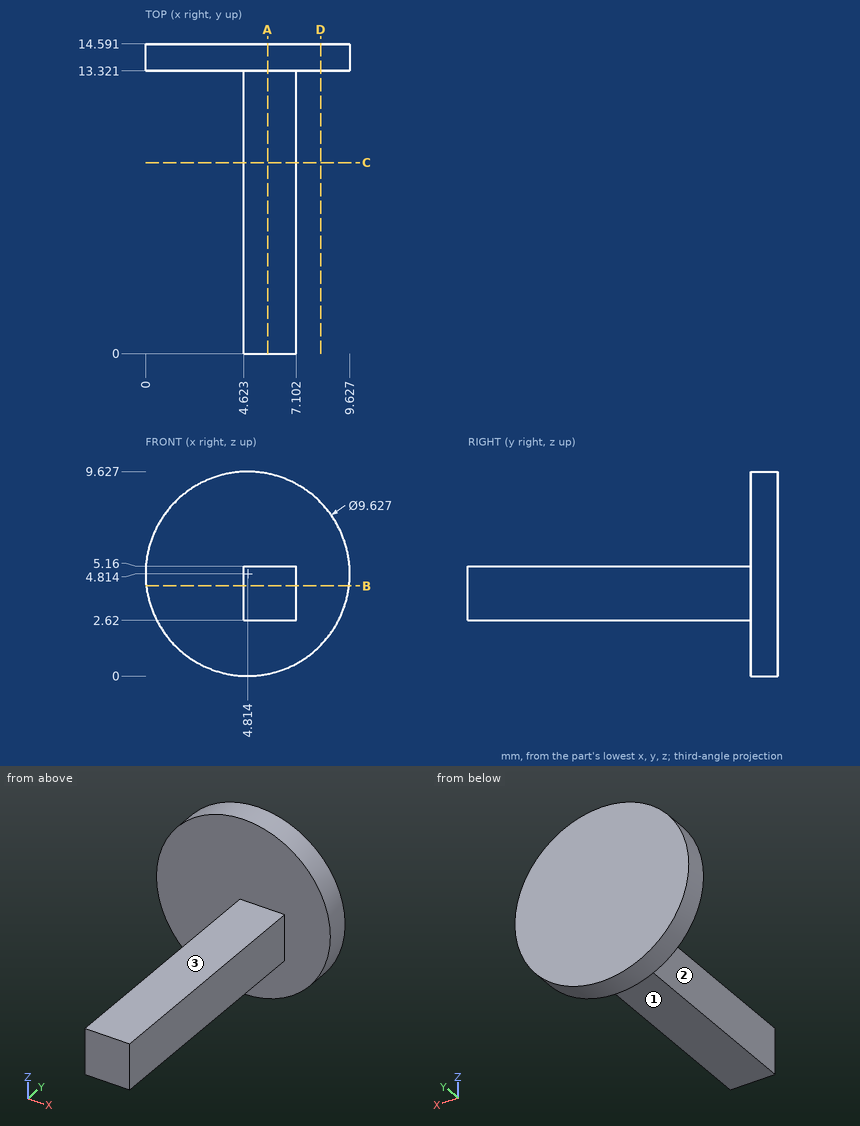
Job drawing, mm, ordinate dimensions from the low corner. One solid piece. A direction names the side the tool comes from. Round coordinates to 2 decimals unless told otherwise and drop trailing zeros. Loops run counter-clockwise (first coordinate to the right, second up) from the corner with the lowest first, then second, coordinate; pieces in that order, holes last.
Item 1: Cut at A-A, the plane x = 5.75. Give the cut face in (y, z) (1 decimal).
Item 2: Drop flat-ended pins along their axis: P1, Ø0.8, axis at y = 4.5, z = 4.5, coming from the +X side; P2, Ø2, axis at x = 6.5, y = 9, coming from the +Z side; P3, Ø4, axis at y = 7, z = 8, coming from the +X side; P4, Ø4, axis at y = 12, z = 2.5, coming from the -X side. Give the stop position or say it passes through.
Item 3: Cut at D-D, the plane x = 8.25. Give the cut face in (y, z) (1 decimal).
Item 4: 3-axis set-ups, long thin cutter, end or side, ignore diameter. For the marked faces 1, 2 and 3: which of +Z, -Z, +X, -X, +Y, -Y reach the whole face in a straight line?
Item 5: Drill centre lines: line 1 (Y direction, x = 3.5, z = 2); line 2 (X direction, y = 11.75, z = 4.75); line 3 (Z direction, x = 4.75, y = 12.5). Where is each one in solid material? Low to high.
Item 6: Cut at B-B, the plane z = 4.25. Give the cut face in (x, y) (1 decimal).
Item 7: Cut at C-C, the plane y = 9. Give the cut face in (x, z).
A:
1. outline: (0, 2.6) - (13.3, 2.6) - (13.3, 0.1) - (14.6, 0.1) - (14.6, 9.5) - (13.3, 9.5) - (13.3, 5.2) - (0, 5.2) - close
2. P1: stops at x = 7.1
2. P2: stops at z = 5.16
2. P3: passes through
2. P4: stops at x = 0.07
3. outline: (13.3, 1.4) - (14.6, 1.4) - (14.6, 8.2) - (13.3, 8.2) - close
4. face 1: -Z, +X, -X, -Y
4. face 2: +Z, -Z, -X, -Y
4. face 3: +Z, +X, -X, -Y
5. line 1: y = 13.32 to 14.59
5. line 2: x = 4.62 to 7.1
5. line 3: z = 2.62 to 5.16
6. outline: (0, 13.3) - (4.6, 13.3) - (4.6, 0) - (7.1, 0) - (7.1, 13.3) - (9.6, 13.3) - (9.6, 14.6) - (0, 14.6) - close
7. outline: (4.62, 2.62) - (7.1, 2.62) - (7.1, 5.16) - (4.62, 5.16) - close
